Could you check a few things on this drawing? It's one solid part, dimensions in mm from its lowest x, y, z. A direction names the side the tool comes from. Give positions to 0.01 mm unless a question says otherwise; leave off trailing zeros. Loops run counter-clockwise (first coordinate to the right, second up) from the corner with the lowest first, then second, coordinate; pieces in that order, holes last. Notation, with made-up numbers: (-10, 82.25) - (14, 82.25) arc R15 cw to (14, 95.25) - close; hole circle Ø7 at (83.5, 15.25). An arc over 180 degrees is marked (long way). Return JSON: item names as keys, results as strings. Group by question number.
(1) If we section it at A-A (x = 69.5): Please give me the cut outline in (y, z), then the cut area to 3 significant figures.
(2) On a 3-axis mill with a long thin cutter (end or side, diameter ignored), from which of +Z, -Z, +X, -X, +Y, -Y can I reach the whole of each face in a straight line? I mean the marked faces 1 and 2. Say none if no direction works.
(3) I need wall thicknesses on probe 1 along Z at (x, y) = (42, 67.5); probe 2 along Y at (x, z) = (22.5, 18). Which ranges of each line are inside material? Lowest first, please. Write a range as [from, to].
(4) For P1, Ø23, axis at x = 28, y = 55, coming from the -Z side; P2, Ø4, axis at x = 31.5, z = 12.5, coming from the -Y side, each with a flat end and sliding along its axis, tell me the tip position at first contact or that it passes through.
(5) If we section it at B-B (z = 9): Please give me the cut outline in (x, y).
(6) If we section it at C-C (y = 56): Please give me the cut outline in (x, z), then the cut area to 3 significant figures.
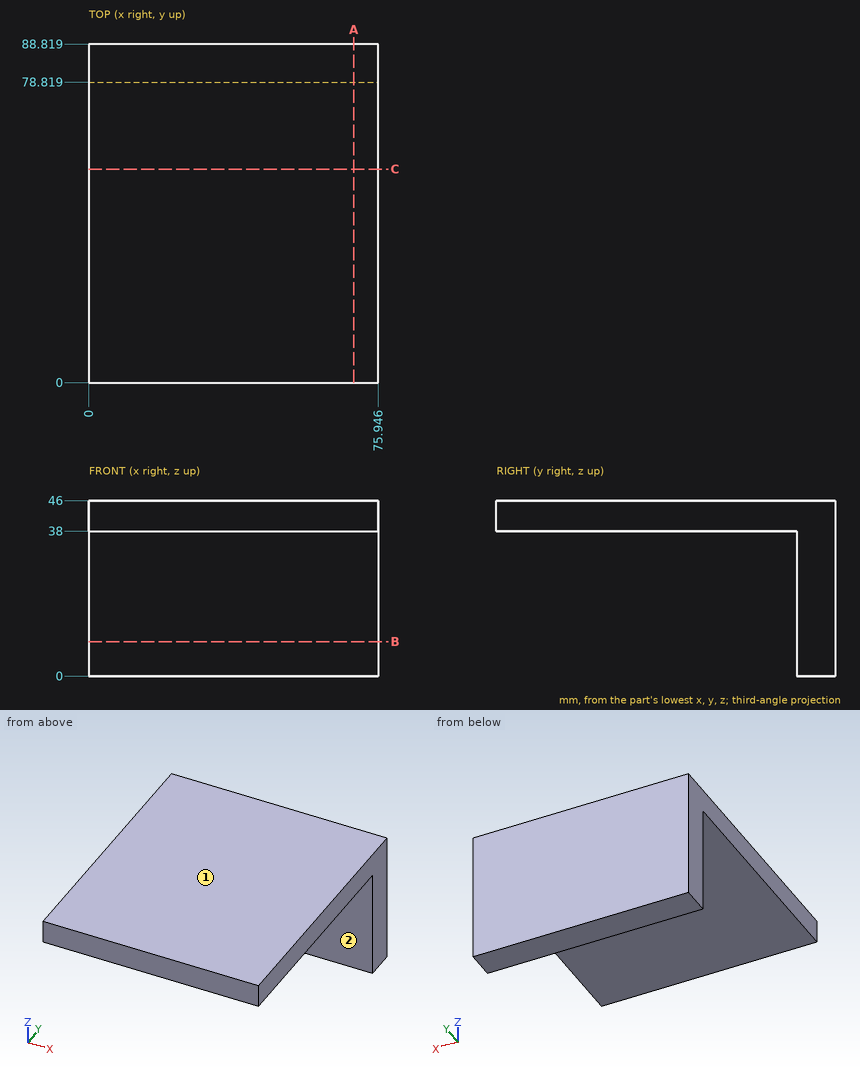
Values:
{
 "1": {"outline": "(0, 38) - (78.82, 38) - (78.82, 0) - (88.82, 0) - (88.82, 46) - (0, 46) - close", "area": "1,090 mm2"},
 "2": {"face 1": "+Z, +X, -X, +Y, -Y", "face 2": "-Z, +X, -X, -Y"},
 "3": {"probe 1": "[38, 46]", "probe 2": "[78.82, 88.82]"},
 "4": {"P1": "z = 38", "P2": "y = 78.82"},
 "5": {"outline": "(0, 78.82) - (75.95, 78.82) - (75.95, 88.82) - (0, 88.82) - close"},
 "6": {"outline": "(0, 38) - (75.95, 38) - (75.95, 46) - (0, 46) - close", "area": "608 mm2"}
}
